```python
from build123d import *

# Parameters (mm, degrees)
BOSS_EXTRUDE1_DEPTH     = 70
CUT_EXTRUDE5_DEPTH      = 24
CUT_EXTRUDE4_DEPTH      = 50
CUT_EXTRUDE4_DEPTH_BACK = 50
SHELL2_T                = -1
FILLET1_R               = 10
CUT_EXTRUDE3_DEPTH      = 26
CUT_EXTRUDE2_DEPTH      = 1
CUT_EXTRUDE2_DEPTH_BACK = 1
SKETCH4_W               = 24
SKETCH4_H               = 6


with BuildPart() as part:
    # Sketch2 → Boss-Extrude1 (new body)
    with BuildSketch(Plane(origin=(0, 0, 0), x_dir=(1, 0, 0), z_dir=(0, 1, 0))):
        Polygon((-18.988562983, 28.382917999), (-4.988562983, 29.470238095), (-1.988562983, 72.470238095), (4.011437017, 72.470238095), (7.011437017, 29.470238095), (32.511437017, 27.489762205), (32.511437017, 20.489762205), (-30.488562983, 20.489762205), (-30.488562983, 27.489762205), align=None)
    extrude(amount=BOSS_EXTRUDE1_DEPTH)

    # Sketch26 → Cut-Extrude5 (cut)
    with BuildSketch(Plane(origin=(0, 70, 0), x_dir=(1, 0, 0), z_dir=(0, 1, 0))):
        Polygon((-4.988562983, 29.470238095), (7.011437017, 29.470238095), (32.511437017, 27.489762205), (32.511437017, 20.489762205), (-30.488562983, 20.489762205), (-30.488562983, 27.489762205), align=None)
    extrude(amount=-CUT_EXTRUDE5_DEPTH, mode=Mode.SUBTRACT)

    # Sketch7 → Cut-Extrude4 (cut, two sides: drawn at the far end of the back side and taken through both)
    with BuildSketch(Plane(origin=(0, 0, 0), x_dir=(0, 0, -1), z_dir=(1, 0, 0)).offset(-CUT_EXTRUDE4_DEPTH_BACK)):
        Polygon((20.489762205, 65), (50.489762205, 70), (20.489762205, 70), align=None)
        Polygon((72.470238095, 63), (50.489762205, 70), (72.470238095, 70), align=None)
    extrude(amount=CUT_EXTRUDE4_DEPTH + CUT_EXTRUDE4_DEPTH_BACK, mode=Mode.SUBTRACT)

    # Shell2
    shell2_openings = [part.faces().sort_by_distance(p)[0] for p in [
        (1.011437017, 0, -34.888692943),
    ]]
    offset(amount=SHELL2_T, openings=shell2_openings, kind=Kind.INTERSECTION)

    # Fillet1
    fillet1_edges = [part.edges().sort_by_distance(p)[0] for p in [
        (1.011437017, 70, -50.489762205),
    ]]
    fillet(fillet1_edges, radius=FILLET1_R)

    # Sketch6 → Cut-Extrude3 (cut)
    with BuildSketch(Plane.XZ):
        Polygon((-4.988562983, -29.470238095), (7.011437017, -29.470238095), (4.011437017, -72.470238095), (-1.988562983, -72.470238095), align=None)
    extrude(amount=-CUT_EXTRUDE3_DEPTH, mode=Mode.SUBTRACT)

    # Sketch4 → Cut-Extrude2 (cut, two sides: drawn at the far end of the back side and taken through both)
    with BuildSketch(Plane(origin=(0, 45, 0), x_dir=(1, 0, 0), z_dir=(0, 1, 0)).offset(-CUT_EXTRUDE2_DEPTH_BACK)):
        Polygon((-29.488562983, 26.596606412), (-17.988562983, 27.489762205), (-17.988562983, 21.489762205), (-29.488562983, 21.489762205), align=None)
        Polygon((31.511437017, 21.489762205), (20.011437017, 21.489762205), (20.011437017, 27.489762205), (31.511437017, 26.596606412), align=None)
        with Locations((7.011437017, 24.489762205)):
            Rectangle(SKETCH4_W, SKETCH4_H)
    extrude(amount=CUT_EXTRUDE2_DEPTH + CUT_EXTRUDE2_DEPTH_BACK, mode=Mode.SUBTRACT)


solid = part.part
```
The listing builds one solid part. Answer for the finished solid, in the listing's coordinates (mm). A direction names the side the tool comes from. Coordinates: 2 decimals unless noted, no trailing zeros. Write each loop counter-clockwise with the first axis right and the second up, starting at its lowest first coordinate (ties: lowest second). Pieces come first, ordered by that corner, then holes. Notation, with made-up numbers: M 6,69.5 L 26,69.5 A8 cw 26,73.5 Z; hole C -26,4 d6. An arc over 180 degrees is marked long. Use a Markdown table: item, result. Add a question column.
1. For a pull along X with two mould halves and no side action, classify faces 5 (the flat face through (1, 23, -20.49)), 6 (the flat face through (-3.51, 47.56, -50.67)), 7 (the flat face through (0.962, 65.575, -61.091)) as +X half, -X half, draft (parallel to the pull), parting line (faces both ways), or undercut.
2. Section B-B (y = 21) is taken. Give the vertices of the cut face in (x, z), plus the area to 3 significant figures.
3. Given P1, Ø4, axis at x = 3, z = -61.5, coming from the +Y side; P2, Ø6, axis at y = 56.5, z = -41, coming from the -X side; P3, Ø10, axis at x = 1.5, z = -27, coming from the +Y side, each flat-ended and moving along its own axis, determine where each tip first touches the part or whether it passes through.
4. Which of the six approach directions +Z, -Z, +X, -X, +Y, -Y give full straight-line access (tool end or side, diameter ignored) to faces 1 (the flat face through (1, 56, -29.47)), 2 (the flat face through (-2.574, 41.668, -49.705)), 3 (the flat face through (-29.489, 23, -24)), 4 (the flat face through (1, 44, -72.47))?
5. Section A-A (y = 50) is taken. Give the vertices of the cut face in (x, z), plus the area to 3 significant figures.
6. Section D-D (z = -45) is taken. Give the vertices of the cut face in (x, y), plus the area to 3 significant figures.
7. Section C-C (x = 16) is taken. Give the vertices of the cut face in (y, z), plus the area to 3 significant figures.
8. Straight lines are drawn through the part: line 1 along Z through (x, y) = (3, 48.5); line 2 along Z through (x, y) = (17.5, 29.5); line 3 along X through (y, z) = (41.5, -23.5). For each, find the intervals that lie inside material, in ascending order. Write a range as [from, to].
Data:
| question | item | result |
|---|---|---|
| 1 | face 5 | draft |
| 1 | face 6 | -X half |
| 1 | face 7 | undercut |
| 2 | outline | M -30.49,-27.49 L -4.99,-29.47 L -3.99,-29.47 L -4.05,-28.54 L -29.49,-26.56 L -29.49,-21.49 L 31.51,-21.49 L 31.51,-26.56 L 6.07,-28.54 L 6.01,-29.47 L 7.01,-29.47 L 32.51,-27.49 L 32.51,-20.49 L -30.49,-20.49 Z |
| 2 | area | 126 mm2 |
| 3 | P1 | stops at y = 67.13 |
| 3 | P2 | stops at x = -4.39 |
| 3 | P3 | stops at y = 66.92 |
| 4 | face 1 | +Z, +X, -X, +Y |
| 4 | face 2 | -Y |
| 4 | face 3 | +Y, -Y |
| 4 | face 4 | -Z, +X, -X, +Y, -Y |
| 5 | outline | M -4.99,-29.47 L -1.99,-72.47 L 4.01,-72.47 L 7.01,-29.47 Z; hole M -3.92,-30.47 L -1.06,-71.47 L 3.08,-71.47 L 5.94,-30.47 Z |
| 5 | area | 100 mm2 |
| 6 | outline | M -3.91,26 L -2.9,26 L -2.9,68.07 L 4.93,68.07 L 4.93,26 L 5.93,26 L 5.93,69.09 L -3.91,69.09 Z |
| 6 | area | 94.3 mm2 |
| 7 | outline | M 0,-28.77 L 46,-28.77 L 46,-27.49 L 45,-27.49 L 45,-27.77 L 0,-27.77 Z; M 0,-21.49 L 46,-21.49 L 46,-20.49 L 0,-20.49 Z |
| 7 | area | 92.4 mm2 |
| 8 | line 1 | z = [-72.47, -71.47], [-30.47, -29.47] |
| 8 | line 2 | z = [-28.66, -27.65], [-21.49, -20.49] |
| 8 | line 3 | x = [-30.49, -29.49], [31.51, 32.51] |
